Could you check a few things on this drawing? It's one solid part, dimensions in mm from its lowest x, y, z. A direction names the side the tool comes from. Give positions to 0.01 mm unless a question says otherwise; leave off trailing zeros. Return JSON: item names as keys, results as strings. Group by question number.
(1) I need wall thicknesses on probe 1 along Y at (x, z) = (102, 237). Which ranges of the line are inside material? Lowest first, please. Write a range as [from, to].
(2) On a 3-axis mill with a long thin cutter (end or side, diameter ignored), from which of +Z, -Z, +X, -X, +Y, -Y can I reach the whole of each face in a straight line? I mean the marked faces 1 and 2. Say none if no direction works.
(3) For P1, Ø7, axis at x = 380.5, z = 138, coming from the -Y side; P2, Ø10, axis at x = 212, z = 285, coming from the -Y side, each with a flat end and sliding along its axis, tell me the tip position at first contact or that it passes through.
(4) If we mould it in two halves opening along X, with no side actions, what happens to the marked faces 3, 4 and 5? For each: released by +X, released by -X, zero draft, split by the parting line, or undercut.
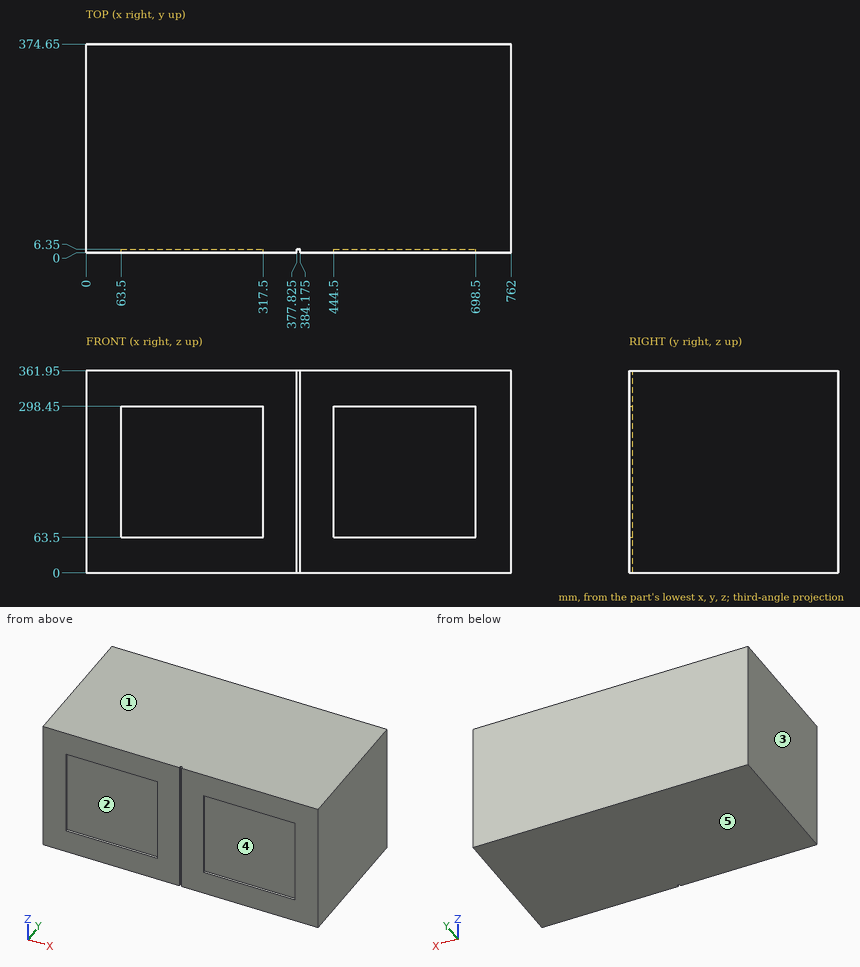
Values:
{
 "1": {"probe 1": "[6.35, 374.65]"},
 "2": {"face 1": "+Z, +X, -X, +Y, -Y", "face 2": "-Y"},
 "3": {"P1": "y = 0", "P2": "y = 6.35"},
 "4": {"face 3": "released by -X", "face 4": "undercut", "face 5": "zero draft"}
}
